Geometry check sheet. Reference: the model listing, model coordinates, mm. A direction names the side the tool comes from. Round coordinates to 2 decimals unless told otherwise and drop trailing zeros. Order: outer loops, then holes, each group sorted by start corner. A loop starts at its lowest first (then second) coordinate and runs counter-clockwise, first axis right, second up.
(1) Sectioned sample at B-B (z = -3.5). Record the boundary of the cut face in (x, y), plus the area to 3 significant figures.
(2) Release check for a two-part mould opening along Y. For faces 1 (the face through (9.76, 2.17, -12.4)), 2 (the face through (61, 0, 0)), 3 (the face through (0.06, -5.75, -2.46)), 4 (the face through (0, -7, -5)) record: +Y half, -Y half, draft (parallel to the pull), parting line (faces both ways), or undercut.
(3) Go/stop test with flat-tipped pins: pin 1 (2 mm diameter, centred on x = 0.5, y = -0.5, fed in from +Z); pin 2 (2 mm diameter, centred on x = -6.999, y = -0.001, fed in from +Z); pin 3 (1 mm diameter, centred on x = 65.5, y = -12.5, fed in from -Z); pin 4 (10 mm diameter, centred on y = -2.5, z = -14.5, fed in from -X). Record where each tip stops, or that it passes through.
(4) Sectioned sample at C-C (y = -16). Record the boundary of the cut face in (x, z), plus the area to 3 significant figures.
(5) Set-up check for faces 5 (the face through (-20, 0, -3)), 6 (the face through (-7, 0, -5)): record each of +Z, -Z, +X, -X, +Y, -Y from which the full face is reachable in a straight line by a thin tool's end or side.
(6) Material ranges on line 1 along X through (y, z) = (-8, -1.75); line 2 along X through (y, z) = (-7, -3.65) (3 decimals); line 3 along Z through (x, y) = (118, -11.5), recorded low to high.
(7) Sectioned sample at D-D (z = -15.75). Record the boundary of the cut face in (x, y).
(8) Sectioned sample at A-A (x = 117). Record the boundary of the cut face in (y, z).
from build123d import *

# Parameters (mm, degrees)
BOSS_EXTRUDE1_DEPTH   = 5
CUT_EXTRUDE1_REACH    = 143.51
SKETCH2_R             = 1
SKETCH2_R_2           = 1.25
CUT_EXTRUDE2_REACH    = 143.51
SKETCH3_R             = 10
BODY_MOVE_COPY1_ANGLE = 90
SKETCH12_R            = 10
BOSS_EXTRUDE2_DEPTH   = 15


with BuildPart() as part:
    # Sketch1 → Boss-Extrude1 (new body)
    with BuildSketch(Plane(origin=(0, 0, 0), x_dir=(1, 0, 0), z_dir=(0, 1, 0))):
        with BuildLine():
            Line((120, -20), (0, -20))
            ThreePointArc((0, -20), (-20, 0), (0, 20))
            Line((0, 20), (120, 20))
            ThreePointArc((120, 20), (140, 0), (120, -20))
        make_face()
    extrude(amount=BOSS_EXTRUDE1_DEPTH)

    # Sketch2 → Cut-Extrude1 (cut, up to next)
    with BuildSketch(Plane(origin=(0, 5, 0), x_dir=(1, 0, 0), z_dir=(0, 1, 0)), mode=Mode.PRIVATE) as cut_extrude1_sk1:
        with Locations(Location((0, 0, 0), (0, 0, 270))):
            Circle(SKETCH2_R)
    cut_extrude1_tool1 = extrude(cut_extrude1_sk1.sketch, amount=-CUT_EXTRUDE1_REACH, mode=Mode.PRIVATE) & part.part
    # Sketch2 → Cut-Extrude1 (cut, up to next)
    with BuildSketch(Plane(origin=(0, 5, 0), x_dir=(1, 0, 0), z_dir=(0, 1, 0)), mode=Mode.PRIVATE) as cut_extrude1_sk2:
        with Locations(Location((0, 7, 0), (0, 0, 270))):
            Circle(SKETCH2_R_2)
    cut_extrude1_tool2 = extrude(cut_extrude1_sk2.sketch, amount=-CUT_EXTRUDE1_REACH, mode=Mode.PRIVATE) & part.part
    # Sketch2 → Cut-Extrude1 (cut, up to next)
    with BuildSketch(Plane(origin=(0, 5, 0), x_dir=(1, 0, 0), z_dir=(0, 1, 0)), mode=Mode.PRIVATE) as cut_extrude1_sk3:
        with Locations(Location((7.001, 0.001, 0), (0, 0, 270))):
            Circle(SKETCH2_R_2)
    cut_extrude1_tool3 = extrude(cut_extrude1_sk3.sketch, amount=-CUT_EXTRUDE1_REACH, mode=Mode.PRIVATE) & part.part
    # Sketch2 → Cut-Extrude1 (cut, up to next)
    with BuildSketch(Plane(origin=(0, 5, 0), x_dir=(1, 0, 0), z_dir=(0, 1, 0)), mode=Mode.PRIVATE) as cut_extrude1_sk4:
        with Locations(Location((0.002, -7, 0), (0, 0, 270))):
            Circle(SKETCH2_R_2)
    cut_extrude1_tool4 = extrude(cut_extrude1_sk4.sketch, amount=-CUT_EXTRUDE1_REACH, mode=Mode.PRIVATE) & part.part
    # Sketch2 → Cut-Extrude1 (cut, up to next)
    with BuildSketch(Plane(origin=(0, 5, 0), x_dir=(1, 0, 0), z_dir=(0, 1, 0)), mode=Mode.PRIVATE) as cut_extrude1_sk5:
        with Locations(Location((-6.999, -0.001, 0), (0, 0, 270))):
            Circle(SKETCH2_R_2)
    cut_extrude1_tool5 = extrude(cut_extrude1_sk5.sketch, amount=-CUT_EXTRUDE1_REACH, mode=Mode.PRIVATE) & part.part
    add(cut_extrude1_tool1.solids().sort_by_distance((0, 5, 0))[0], mode=Mode.SUBTRACT)
    add(cut_extrude1_tool2.solids().sort_by_distance((0, 5, -7))[0], mode=Mode.SUBTRACT)
    add(cut_extrude1_tool3.solids().sort_by_distance((7.001, 5, -0.001))[0], mode=Mode.SUBTRACT)
    add(cut_extrude1_tool4.solids().sort_by_distance((0.002, 5, 7))[0], mode=Mode.SUBTRACT)
    add(cut_extrude1_tool5.solids().sort_by_distance((-6.999, 5, 0.001))[0], mode=Mode.SUBTRACT)

    # Sketch3 → Cut-Extrude2 (cut, up to next)
    with BuildSketch(Plane(origin=(0, 5, 0), x_dir=(1, 0, 0), z_dir=(0, 1, 0)), mode=Mode.PRIVATE) as cut_extrude2_sk1:
        with Locations(Location((120, 0, 0), (0, 0, 270))):
            Circle(SKETCH3_R)
    cut_extrude2_tool1 = extrude(cut_extrude2_sk1.sketch, amount=-CUT_EXTRUDE2_REACH, mode=Mode.PRIVATE) & part.part
    add(cut_extrude2_tool1.solids().sort_by_distance((120, 5, 0))[0], mode=Mode.SUBTRACT)


with BuildPart() as part_1:
    # Body-Move/Copy1: moved
    add(part.part.rotate(Axis((0, 0, 0), (1, 0, 0)), BODY_MOVE_COPY1_ANGLE))

    # Sketch12 → Boss-Extrude2 (add)
    with BuildSketch(Plane(origin=(0, 0, 0), x_dir=(-1, 0, 0), z_dir=(0, 0, -1))):
        with Locations(Location((0, 0, 0), (0, 0, 270))):
            Circle(SKETCH12_R)
    extrude(amount=BOSS_EXTRUDE2_DEPTH)


with BuildPart() as part_2:
    # Body-Move/Copy4: moved
    add(part_1.part.moved(Location((0, 0, -5))))


solid = part_2.part
Answer below:
1. outline: (0, -20) - (120, -20) arc R20 ccw to (120, 20) - (0, 20) arc R20 ccw to start; hole circle Ø2.5 at (-7, 0); hole circle Ø2.5 at (0, -7); hole circle Ø2.5 at (0, 7); hole circle Ø2 at (0, 0); hole circle Ø2.5 at (7, 0); hole circle Ø20 at (120, 0)
1. area: 5,720 mm2
2. face 1: parting line
2. face 2: draft
2. face 3: undercut
2. face 4: undercut
3. pin 1: stops at z = 0
3. pin 2: stops at z = -5
3. pin 3: stops at z = -5
3. pin 4: stops at x = -10
4. outline: (-12, -5) - (132, -5) - (132, 0) - (-12, 0) - close
4. area: 720 mm2
5. face 5: +Z, -Z, -X
5. face 6: +Z
6. line 1: x = -18.33 to -0.75, 0.75 to 114, 126 to 138.33
6. line 2: x = -18.735 to -1.248, 1.252 to 112.859, 127.141 to 138.735
6. line 3: z = -5 to 0
7. outline: circle Ø20 at (0, 0)
8. outline: (-20, -5) - (-9.54, -5) - (-9.54, 0) - (-20, 0) - close; (9.54, -5) - (20, -5) - (20, 0) - (9.54, 0) - close
